Check sheet for the modelled part. Datum: model origin and axes. Units: mm. A direction names the side the tool comes from. Round coordinates to 2 decimals unless told otherwise and drop trailing zeros. Order: outer loops, then holes, each group sorted by start corner. A loop starts at its lowest first (then second) coordinate and runs counter-clockwise, first axis right, second up. Notation, with made-up numbers: (46, 29.25) -> (98, 29.25) arc R15 ccw to (98, 51.25) -> close; hole circle Ø1 at (23, 64). An arc over 180 degrees is marked (long way). Use CSV: the item, a comma, the result in double quotes.
```python
from build123d import *

# Parameters (mm, degrees)
BOSS_EXTRUDE2_DEPTH = 109.3
SKETCH4_W           = 14.8
SKETCH4_H           = 19
BOSS_EXTRUDE3_DEPTH = 11
SKETCH5_W           = 14.8
SKETCH5_H           = 20
BOSS_EXTRUDE4_DEPTH = 25.4
SKETCH7_W           = 14.8
SKETCH7_H           = 20
BOSS_EXTRUDE5_DEPTH = 1.4
SKETCH8_W           = 7.8
SKETCH8_H           = 4.5
BOSS_EXTRUDE6_DEPTH = 7.8
SKETCH9_R           = 2
CUT_EXTRUDE1_DEPTH  = 156.666149178
FILLET1_R           = 2.25
SKETCH10_R          = 0.25
CUT_EXTRUDE2_DEPTH  = 156.95928956


with BuildPart() as part:
    # Sketch3 → Boss-Extrude2 (new body)
    with BuildSketch(Plane.XY):
        with BuildLine():
            Line((-6, -5.291502622), (-6, 5.291502622))
            ThreePointArc((-6, 5.291502622), (0, 8), (6, 5.291502622))
            Line((6, 5.291502622), (6, -5.291502622))
            ThreePointArc((6, -5.291502622), (0, -8), (-6, -5.291502622))
        make_face()
        with BuildLine():
            Line((-3.05, -3.308700651), (-3.05, 3.308700651))
            ThreePointArc((-3.05, 3.308700651), (0, 4.5), (3.05, 3.308700651))
            Line((3.05, 3.308700651), (3.05, -3.308700651))
            ThreePointArc((3.05, -3.308700651), (0, -4.5), (-3.05, -3.308700651))
        make_face(mode=Mode.SUBTRACT)
    extrude(amount=BOSS_EXTRUDE2_DEPTH)

    # Sketch4 → Boss-Extrude3 (add)
    with BuildSketch(Plane.XY.offset(109.3)):
        Rectangle(SKETCH4_W, SKETCH4_H)
        with BuildLine():
            Line((-3.05, 3.308700651), (-3.05, -3.308700651))
            ThreePointArc((-3.05, -3.308700651), (0, -4.5), (3.05, -3.308700651))
            Line((3.05, -3.308700651), (3.05, 3.308700651))
            ThreePointArc((3.05, 3.308700651), (0, 4.5), (-3.05, 3.308700651))
        make_face(mode=Mode.SUBTRACT)
    extrude(amount=BOSS_EXTRUDE3_DEPTH)

    # Sketch5 → Boss-Extrude4 (add)
    with BuildSketch(Plane.XY.offset(120.3)):
        with Locations((0, 0.5)):
            Rectangle(SKETCH5_W, SKETCH5_H)
        with BuildLine():
            Line((-3.05, 3.308700651), (-3.05, -3.308700651))
            ThreePointArc((-3.05, -3.308700651), (0, -4.5), (3.05, -3.308700651))
            Line((3.05, -3.308700651), (3.05, 3.308700651))
            ThreePointArc((3.05, 3.308700651), (0, 4.5), (-3.05, 3.308700651))
        make_face(mode=Mode.SUBTRACT)
    extrude(amount=BOSS_EXTRUDE4_DEPTH)

    # Sketch7 → Boss-Extrude5 (add)
    with BuildSketch(Plane.XY.offset(145.7)):
        with Locations((0, 0.5)):
            Rectangle(SKETCH7_W, SKETCH7_H)
    extrude(amount=BOSS_EXTRUDE5_DEPTH)

    # Sketch8 → Boss-Extrude6 (add)
    with BuildSketch(Plane.XY.offset(147.1)):
        with Locations((0, 0.5)):
            Rectangle(SKETCH8_W, SKETCH8_H)
    extrude(amount=BOSS_EXTRUDE6_DEPTH)

    # Sketch9 → Cut-Extrude1 (cut, through all)
    with BuildSketch(Plane.ZY.offset(3.9)):
        with Locations((150.4, 0.5)):
            Circle(SKETCH9_R)
    extrude(amount=-CUT_EXTRUDE1_DEPTH, mode=Mode.SUBTRACT)

    # Fillet1
    fillet1_edges = [part.edges().sort_by_distance(p)[0] for p in [
        (0, -1.75, 154.9),
        (0, 2.75, 154.9),
    ]]
    fillet(fillet1_edges, radius=FILLET1_R - 0.0001)  # a hair under: the kernel refuses the full size

    # Sketch10 → Cut-Extrude2 (cut, through all)
    with BuildSketch(Plane.ZY.offset(7.4)):
        with Locations((120.7, -6.6)):
            Circle(SKETCH10_R)
        with Locations((146.7, -6.6)):
            Circle(SKETCH10_R)
        with Locations((120.7, 10.1)):
            Circle(SKETCH10_R)
        with Locations((146.7, 10.1)):
            Circle(SKETCH10_R)
    extrude(amount=-CUT_EXTRUDE2_DEPTH, mode=Mode.SUBTRACT)


solid = part.part
```
Q1. Mould release check, pull along Z, two halves, no side actions. Record for faces 6 (the face through (-0.055, -0.266, 152.247)), 7 (the face through (0, 0, 145.7)), 8 (the face through (0, -4.5, 71.8)): pulls with the +Z half, pulls with the -Z half, needs draft (parallel to the pull), parting line crosses it, or undercut.
Result sheet:
face 6,"undercut"
face 7,"pulls with the -Z half"
face 8,"needs draft"
Q2. Go/stop test with flat-tipped pins: pin 1 (5 mm diameter, centred on x = 4.5, y = -5.5, fed in from -Z); pin 2 (3.5 mm diameter, centred on y = 0.5, z = 91, fed in from +X); pin 3 (2 mm diameter, centred on y = -0.5, z = 36.5, fed in from -X); pin 4 (3 mm diameter, centred on x = 3.5, z = 93.5, fed in from +Y). Record where each tip stops, or that it passes through.
Result sheet:
pin 1,"stops at z = 0"
pin 2,"stops at x = 6"
pin 3,"stops at x = -6"
pin 4,"stops at y = 7.75"
Q3. Sectioned sample at A-A, the plane z = 150.4. Enter the section's corners in (x, y), then the cut area to 3 significant figures.
Result sheet:
outline,"(-3.9, -1.75) -> (3.9, -1.75) -> (3.9, -1.5) -> (-3.9, -1.5) -> close; (-3.9, 2.5) -> (3.9, 2.5) -> (3.9, 2.75) -> (-3.9, 2.75) -> close"
area,"3.90 mm^2"
Q4. Scan lines: L1, parallel to Y at x = 2.5, z = 146.7; L2, parallel to Y at x = 2.25, z = 120.7; L3, parallel to X at y = 2, z = 43.5. Record each from-to range of solid material in increasing order.
Result sheet:
L1,"y = -9.5 to -6.85, -6.35 to 9.85, 10.35 to 10.5"
L2,"y = -9.5 to -6.85, -6.35 to -3.9, 3.9 to 9.85, 10.35 to 10.5"
L3,"x = -6 to -3.05, 3.05 to 6"
Q5. Sectioned sample at C-C, the plane z = 128. Enter the section's corners in (x, y), then the cut area to 3 significant figures.
Result sheet:
outline,"(-7.4, -9.5) -> (7.4, -9.5) -> (7.4, 10.5) -> (-7.4, 10.5) -> close; hole (-3.05, -3.31) arc R4.5 ccw to (3.05, -3.31) -> (3.05, 3.31) arc R4.5 ccw to (-3.05, 3.31) -> close"
area,"246 mm^2"
Q6. Access from +Z, -Z, +X, -X, +Y, -Y to the whole of each face (thin tool, end or side, straight path). Record for faces 1 (the face through (6, 0, 54)), 2 (the face through (0, 9.5, 115)), 3 (the face through (0, -8, 54)), 4 (the face through (0, 8, 54)), 5 (the face through (-7, 0, 109.3)).
Result sheet:
face 1,"-Z, +X, +Y, -Y"
face 2,"-Z, +X, -X, +Y"
face 3,"-Z, -Y"
face 4,"-Z, +Y"
face 5,"-Z"
Q7. Sectioned sample at B-B, the plane z = 87. Enter the section's corners in (x, y).
Result sheet:
outline,"(-6, -5.29) arc R8 ccw to (6, -5.29) -> (6, 5.29) arc R8 ccw to (-6, 5.29) -> close; hole (-3.05, -3.31) arc R4.5 ccw to (3.05, -3.31) -> (3.05, 3.31) arc R4.5 ccw to (-3.05, 3.31) -> close"
